```python
from build123d import *

# Parameters (mm, degrees)
PAD005_DEPTH    = 8.1
POCKET003_DEPTH = 7
SKETCH010_W     = 6.8
SKETCH010_H     = 5
POCKET004_DEPTH = 1
SKETCH011_W     = 5.5
SKETCH011_H     = 3
POCKET005_DEPTH = 3
PAD006_DEPTH    = 4
PAD007_DEPTH    = 0.5


with BuildPart() as part:
    # Sketch008 → Pad005 (new body)
    with BuildSketch(Plane.XY):
        Polygon((-5, 0), (-3.05, 0), (-3.05, 1), (3.05, 1), (3.05, 0), (5, 0), (5, 5.1), (-5, 5.1), align=None)
    extrude(amount=PAD005_DEPTH)

    # Sketch009 (on Face10 of Pad005) → Pocket003 (cut)
    with BuildSketch(Plane.XY.offset(8.1)):
        Polygon((-4.45, 0.55), (-3.45, 0.55), (-3.45, 1.55), (3.45, 1.55), (3.45, 0.55), (4.45, 0.55), (4.45, 4.55), (-4.45, 4.55), align=None)
    extrude(amount=-POCKET003_DEPTH, mode=Mode.SUBTRACT)

    # Sketch010 (on Face5 of Pocket003) → Pocket004 (cut)
    with BuildSketch(Plane.XY.offset(8.1)):
        with Locations((0, 5.5)):
            Rectangle(SKETCH010_W, SKETCH010_H)
    extrude(amount=-POCKET004_DEPTH, mode=Mode.SUBTRACT)

    # Sketch011 (on Face5 of Pocket004) → Pocket005 (cut)
    with BuildSketch(Plane.XY.offset(8.1)):
        with Locations((0, 1.5)):
            Rectangle(SKETCH011_W, SKETCH011_H)
    extrude(amount=-POCKET005_DEPTH, mode=Mode.SUBTRACT)

    # Sketch012 (on Face26 of Pocket005) → Pad006 (join)
    with BuildSketch(Plane.XY.offset(1.1)):
        with BuildLine():
            ThreePointArc((-3.4, 3.25), (-3.65, 3), (-3.4, 2.75))
            Line((-3.4, 2.75), (3.4, 2.75))
            ThreePointArc((3.4, 2.75), (3.65, 3), (3.4, 3.25))
            Line((-3.4, 3.25), (3.4, 3.25))
        make_face()
    extrude(amount=PAD006_DEPTH)

    # Sketch013 → Pad007 (join)
    with BuildSketch(Plane.XY):
        with BuildLine():
            ThreePointArc((-3, 3.75), (-3.75, 3), (-3, 2.25))
            Line((-3, 2.25), (3, 2.25))
            ThreePointArc((3, 2.25), (3.75, 3), (3, 3.75))
            Line((-3, 3.75), (3, 3.75))
        make_face()
    extrude(amount=-PAD007_DEPTH)


with BuildPart() as part_1:
    # Body005 placement: moved
    add(part.part.moved(Location((0.2, 3.4, 1.6))))


solid = part_1.part
```
The model under review builds one solid part; all positions refer to its coordinate system, in mm. A direction names the side the tool comes from. Round coordinates to 2 decimals unless told otherwise and drop trailing zeros. Loops run counter-clockwise (first coordinate to the right, second up) from the corner with the lowest first, then second, coordinate; pieces in that order, holes last. Notation, with made-up numbers: (8, -0.5) -> (16, -0.5) arc R12 cw to (16, 18.5) -> close; hole circle Ø3 at (-27, 54). An arc over 180 degrees is marked (long way). Answer as a JSON object with one key per item and string values. Group by question number.
1) We need section A-A on z = 6.5. Write out the cut boundary in (x, y), then the cut area to 3 significant figures.
2) For faces 1 (the face through (3.25, 4, 6)), 2 (the face through (-4.8, 6, 6)), 3 (the face through (4.65, 6, 6)), list the 3-axis set-ups (+Z, -Z, +X, -X, +Y, -Y) from which the entire face can be reached by the end or side of a thin tool; tool diameter is ignored.
3) We need section C-C on x = 1.5. Write out the cut boundary in (y, z), then the cut area to 3 significant figures.
4) For pin 1 Ø3 at (x, z) = (1, 6.5) entering from -Y; pin 2 Ø0.6 at (x, y) = (1, 4.5) entering from +Z; pin 3 Ø1.5 at (x, y) = (2.5, 5) entering from +Z, all flat-tipped, find the tip position at first contact; note any pin that passes through.
5) We need section D-D on z = 2.25. Write out the cut boundary in (x, y).
6) Mouldability with a two-part tool opening along Y and no side actions: class faces 4 (the face through (0, 7.95, 6)), 5 (the face through (0, 5, 1.6)), 6 (the face through (0, 8.5, 6)) as released by +Y, released by -Y, zero draft, split by the parting line, or undercut.
7) For line 1 (X direction, y = 4.25, z = 3.5); line 2 (Y direction, x = -2.25, z = 4.75); line 3 (X direction, y = 4.55, z = 4), list the stretches that pass through material, from the lowest coordinate up. Write a range as [from, to].
8) We need section B-B on y = 6.85. Write out the cut boundary in (x, z).
Result set:
{
 "1": {"outline": "(-4.8, 3.4) -> (-2.85, 3.4) -> (-2.85, 4.4) -> (3.25, 4.4) -> (3.25, 3.4) -> (5.2, 3.4) -> (5.2, 8.5) -> (-4.8, 8.5) -> close; (-3.2, 6.15) -> (3.6, 6.15) arc R0.25 ccw to (3.6, 6.65) -> (-3.2, 6.65) arc R0.25 ccw to start; hole (-4.25, 3.95) -> (-3.25, 3.95) -> (-3.25, 4.95) -> (3.65, 4.95) -> (3.65, 3.95) -> (4.65, 3.95) -> (4.65, 7.95) -> (-4.25, 7.95) -> close", "area": "19.8 mm²"},
 "2": {"face 1": "+Z, -Z, -Y", "face 2": "+Z, -Z, -X, +Y, -Y", "face 3": "+Z"},
 "3": {"outline": "(4.4, 1.6) -> (5.65, 1.6) -> (5.65, 1.1) -> (7.15, 1.1) -> (7.15, 1.6) -> (8.5, 1.6) -> (8.5, 8.7) -> (7.95, 8.7) -> (7.95, 2.7) -> (6.65, 2.7) -> (6.65, 6.7) -> (6.15, 6.7) -> (6.15, 2.7) -> (4.95, 2.7) -> (4.95, 6.7) -> (4.4, 6.7) -> close", "area": "12.8 mm²"},
 "4": {"pin 1": "y = 4.4", "pin 2": "z = 6.7", "pin 3": "z = 9.7"},
 "5": {"outline": "(-4.8, 3.4) -> (-2.85, 3.4) -> (-2.85, 4.4) -> (3.25, 4.4) -> (3.25, 3.4) -> (5.2, 3.4) -> (5.2, 8.5) -> (-4.8, 8.5) -> close"},
 "6": {"face 4": "undercut", "face 5": "zero draft", "face 6": "released by +Y"},
 "7": {"line 1": "[-4.8, -4.25], [-3.25, -2.85], [3.25, 3.65], [4.65, 5.2]", "line 2": "[4.4, 4.95], [6.15, 6.65], [7.95, 8.5]", "line 3": "[-4.8, -4.25], [-3.25, 3.65], [4.65, 5.2]"},
 "8": {"outline": "(-4.8, 1.6) -> (-3.4, 1.6) -> (-3.4, 1.1) -> (3.8, 1.1) -> (3.8, 1.6) -> (5.2, 1.6) -> (5.2, 9.7) -> (4.65, 9.7) -> (4.65, 2.7) -> (-4.25, 2.7) -> (-4.25, 9.7) -> (-4.8, 9.7) -> close"}
}
